Input: dimensioned drawing with shaded views. Units: mm. Origin: part minimum x, y, z. A direction names the side the tool comes from. Coordinates: 2 decimals unless noted, no trailing zeros. Order: outer loops, then holes, each group sorted by start corner. A loop starts at its lowest first (then second) coordinate and runs counter-clockwise, first axis right, second up. Notation, with made-up numbers: (-7.75, 10) - (43.25, 10) arc R19 ccw to (43.25, 46) - close; hole circle Ø10 at (-27.75, 84). An arc over 180 degrees is marked (long way). Answer as CSV lines item,"result". Start each with the question number.
Item 1: Section B-B (z = 9.05). Output: boundary loops of the cut face in (x, y).
Item 2: Section D-D (y = 14.5). Output: boundary loops of the cut face in (x, z), and give its area (3 significant figures).
Item 3: Access query for the marked faces 5 and 6. Directions: +Z, -Z, +X, -X, +Y, -Y. A direction counts if a zero-diameter tool reaches every point of the face in a straight line with its end or side. Return the directions, or none.
Item 4: Section C-C (x = 21). Output: boundary loops of the cut face in (y, z).
Item 5: Section A-A (x = 11.5). Output: boundary loops of the cut face in (y, z), and give its area (3 significant figures).
Item 6: First-contact query: pin 1 (10 mm diameter, centred on x = 19, y = 47, fed in from -Z); pin 2 (1.5 mm diameter, centred on x = 21.5, y = 17, fed in from -Z); pin 3 (6 mm diameter, centred on x = 10, z = 9.5, fed in from -Y); pin 4 (1 mm diameter, centred on y = 41.5, z = 8, fed in from -X). Flat tips, straight axial feed; report the tip coordinate or a pass-through.
Item 7: Draft query along Z for the marked faces 1, 2, 3 and 4. Return one class per face: +Z half, -Z half, draft (parallel to the pull), parting line (faces both ways), or undercut.
Item 8: Material intervals for line 1 along Z through (x, y) = (7.25, 87); line 2 along X through (y, z) = (86, 11.75); line 3 along Y through (x, z) = (26.25, 12), sorted ascending.
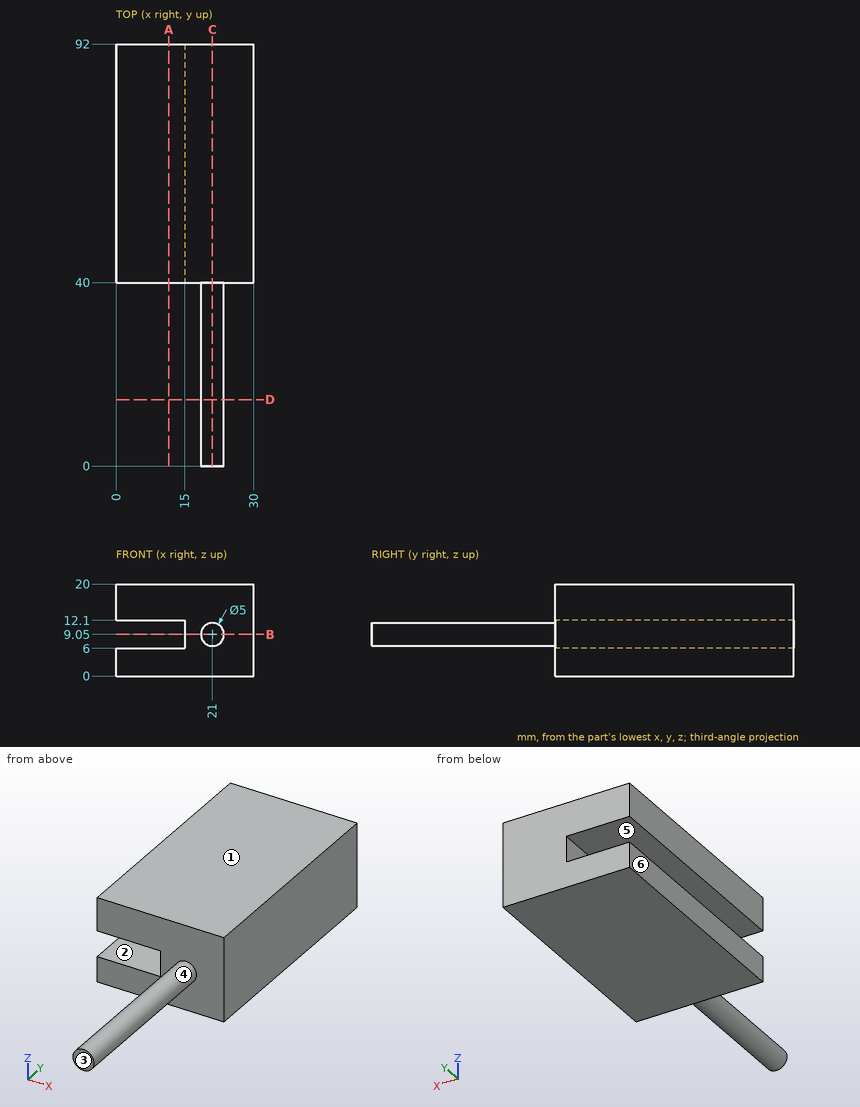
Determined:
1,outline,"(15, 40) - (18.5, 40) - (18.5, 0) - (23.5, 0) - (23.5, 40) - (30, 40) - (30, 92) - (15, 92) - close"
2,outline,"circle Ø5 at (21, 9.05)"
2,area,"19.6 mm^2"
3,face 5,"-X, +Y, -Y"
3,face 6,"+Z, -Z, -X, +Y, -Y"
4,outline,"(0, 6.55) - (40, 6.55) - (40, 0) - (92, 0) - (92, 20) - (40, 20) - (40, 11.55) - (0, 11.55) - close"
5,outline,"(40, 0) - (92, 0) - (92, 6) - (40, 6) - close; (40, 12.1) - (92, 12.1) - (92, 20) - (40, 20) - close"
5,area,"723 mm^2"
6,pin 1,"stops at z = 0"
6,pin 2,"stops at z = 6.55"
6,pin 3,"stops at y = 40"
6,pin 4,"stops at x = 15"
7,face 1,"+Z half"
7,face 2,"undercut"
7,face 3,"draft"
7,face 4,"parting line"
8,line 1,"z = 0 to 6, 12.1 to 20"
8,line 2,"x = 15 to 30"
8,line 3,"y = 40 to 92"
